Can you work these out from the model? Positions are in its coordinate system, mm. Give positions to 0.01 mm unless a question says otherwise; leave off trailing zeros. Order: outer loops, then holes, each group sorted by start corner. A loop starts at its lowest first (then second) coordinate and runs counter-clockwise, first axis right, second up.
```python
from build123d import *

# Parameters (mm, degrees)
SKETCH_1_R      = 2
EXTRUDE_1_DEPTH = 3
FILLET_2_R      = 5
FILLET_3_R      = 5
FILLET_4_R      = 5


with BuildPart() as part:
    # 草图1 → 凸台-拉伸1 (new body)
    with BuildSketch(Plane.XY):
        Polygon((-60, 5), (40, 5), (40, 10), (60, 10), (60, -10), (40, -10), (40, -5), (-60, -5), align=None)
        with Locations((-55.138487595, 0)):
            Circle(SKETCH_1_R, mode=Mode.SUBTRACT)
        with Locations((-40.138487595, 0)):
            Circle(SKETCH_1_R, mode=Mode.SUBTRACT)
        with Locations((50, 0)):
            Circle(SKETCH_1_R, mode=Mode.SUBTRACT)
    extrude(amount=EXTRUDE_1_DEPTH)

    # 圆角2
    fillet_2_edges = [part.edges().sort_by_distance(p)[0] for p in [
        (-60, -5, 1.5),
        (-60, 5, 1.5),
        (60, -10, 1.5),
        (60, 10, 1.5),
    ]]
    fillet(fillet_2_edges, radius=FILLET_2_R - 0.0001)  # a hair under: the kernel refuses the full size

    # 圆角3
    fillet_3_edges = [part.edges().sort_by_distance(p)[0] for p in [
        (40, -5, 1.5),
        (40, 5, 1.5),
    ]]
    fillet(fillet_3_edges, radius=FILLET_3_R - 0.0001)  # a hair under: the kernel refuses the full size

    # 圆角4
    fillet_4_edges = [part.edges().sort_by_distance(p)[0] for p in [
        (40, -10, 1.5),
        (40, 10, 1.5),
    ]]
    fillet(fillet_4_edges, radius=FILLET_4_R)


solid = part.part
```
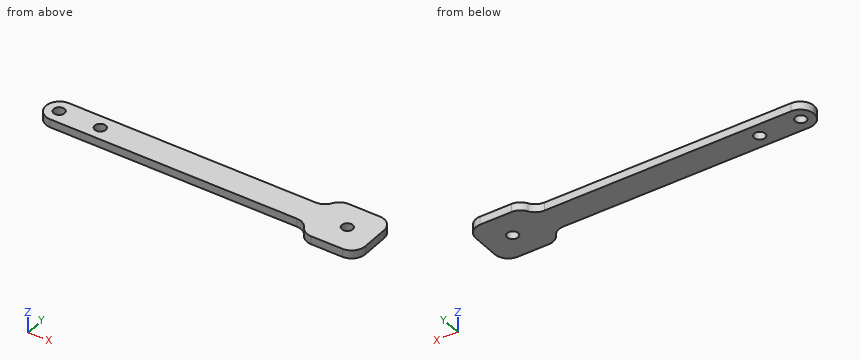
1) I'm going to push flat-ended pins straight in: pin 1 Ø1 at (x, z) = (4.5, 1) entering from -Y; pin 2 Ø1.5 at (y, z) = (4, 0.5) entering from -X; pin 3 Ø1.5 at (x, z) = (2.5, 2) entering from +Y. Where does each tip first touch, or does it pass through?
2) Suppose I cut it at C-C (x = 17). Please give me the cut outline in (y, z), and give its area (3 significant figures).
3) If I drill on line 1 (Y direction, x = -40, z = 2.55); line 2 (Y direction, x = 50, z = 0.8); line 3 (X direction, y = 0.25, z = 1.15), over which ranges is the centre line in solid material (lowest first)?
4) Suppose I cut it at A-A (x = 50). Please give me the cut outline in (y, z), and give its area (3 significant figures).
5) Suppose I cut it at B-B (z = 0.85). Give the number of separate pieces and of enclosed holes in the cut face, and give its area (3 significant figures).
6) Suppose I cut it at D-D (y = 6). Please give me the cut outline in (x, z), and give its area (3 significant figures).
Results:
1. pin 1: stops at y = -5
1. pin 2: stops at x = -58.8
1. pin 3: stops at y = 5
2. outline: (-5, 0) - (5, 0) - (5, 3) - (-5, 3) - close
2. area: 30.0 mm2
3. line 1: y = -5 to -2, 2 to 5
3. line 2: y = -10 to -2, 2 to 10
3. line 3: x = -59.99 to -57.12, -53.15 to -42.12, -38.15 to 48.02, 51.98 to 60
4. outline: (-10, 0) - (-2, 0) - (-2, 3) - (-10, 3) - close; (2, 0) - (10, 0) - (10, 3) - (2, 3) - close
4. area: 48.0 mm2
5. separate pieces: 1
5. enclosed holes: 3
5. area: 1,350 mm2
6. outline: (38, 0) - (59.9, 0) - (59.9, 3) - (38, 3) - close
6. area: 65.7 mm2
